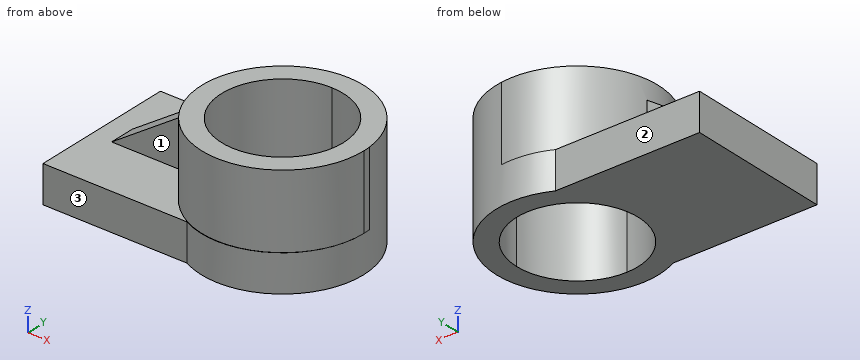
from build123d import *

# Parameters (mm, degrees)
F1_DEPTH = 25.4
F2_DEPTH = 76.2
F4_DEPTH = 50.8
F6_DEPTH = 38.1
F9_DEPTH = 50.8


with BuildPart() as f1:
    # F0 (on Top) → F1 (new body)
    with BuildSketch(Plane.XY):
        with BuildLine():
            ThreePointArc((36.7828311237, -49.6836304665), (6.3025091863, 0), (36.7828311237, 49.6836304665))
            Line((36.7828311237, 49.6836304665), (-62.0354041457, 49.6836304665))
            Line((-62.0354041457, 49.6836304665), (-62.0354041457, -49.6836304665))
            Line((-62.0354041457, -49.6836304665), (36.7828311237, -49.6836304665))
        make_face()
    extrude(amount=F1_DEPTH)

    # F0 (on Top) → F2 (join)
    with BuildSketch(Plane.XY):
        with BuildLine():
            Line((62.0354041457, 41.7620725768), (62.0354041457, 49.6836304665))
            Line((62.0354041457, 49.6836304665), (36.7828311237, 49.6836304665))
            ThreePointArc((36.7828311237, 49.6836304665), (6.3025091863, 0), (36.7828311237, -49.6836304665))
            Line((36.7828311237, -49.6836304665), (62.0354041457, -49.6836304665))
            Line((62.0354041457, -49.6836304665), (62.0354041457, -41.7620725768))
            ThreePointArc((62.0354041457, -41.7620725768), (20.2733315689, 0), (62.0354041457, 41.7620725768))
        make_face()
        with BuildLine():
            Line((36.7828311237, 49.6836304665), (62.0354041457, 49.6836304665))
            Line((62.0354041457, 49.6836304665), (62.0354041457, 41.7620725768))
            ThreePointArc((62.0354041457, 41.7620725768), (91.5656488612, 29.5302447155), (103.7974767226, 0))
            ThreePointArc((103.7974767226, 0), (91.5656488612, -29.5302447155), (62.0354041457, -41.7620725768))
            Line((62.0354041457, -41.7620725768), (62.0354041457, -49.6836304665))
            Line((62.0354041457, -49.6836304665), (36.7828311237, -49.6836304665))
            ThreePointArc((36.7828311237, -49.6836304665), (91.1794994385, -47.5055500981), (117.7682991051, 0))
            ThreePointArc((117.7682991051, 0), (91.1794994385, 47.5055500981), (36.7828311237, 49.6836304665))
        make_face()
        with BuildLine():
            ThreePointArc((36.7828311237, -49.6836304665), (6.3025091863, 0), (36.7828311237, 49.6836304665))
            Line((36.7828311237, 49.6836304665), (-62.0354041457, 49.6836304665))
            Line((-62.0354041457, 49.6836304665), (-62.0354041457, -49.6836304665))
            Line((-62.0354041457, -49.6836304665), (36.7828311237, -49.6836304665))
        make_face()
    extrude(amount=F2_DEPTH)

    # F3 (on face) → F4 (cut)
    with BuildSketch(Plane.XY.offset(76.2)):
        with BuildLine():
            ThreePointArc((117.5399853374, 5.0395483226), (117.7039365392, 2.5789094219), (117.7586227951, 0.1134209896))
            ThreePointArc((117.7586227951, 0.1134209896), (20.3132089265, -36.5094395307), (69.5168613964, 55.2284652871))
            ThreePointArc((69.5168613964, 55.2284652871), (52.7273733531, 54.9501241429), (36.7828311237, 49.6836304665))
            Line((36.7828311237, 49.6836304665), (-62.0354041457, 49.6836304665))
            Line((-62.0354041457, 49.6836304665), (-62.0354041457, -49.6836304665))
            Line((-62.0354041457, -49.6836304665), (36.7828311237, -49.6836304665))
            ThreePointArc((36.7828311237, -49.6836304665), (93.2996420825, -46.1378695519), (117.5399853374, 5.0395483226))
        make_face()
    extrude(amount=-F4_DEPTH, mode=Mode.SUBTRACT)

    # F5 (on face) → F6 (join)
    with BuildSketch(Plane.XY.offset(25.4)):
        with BuildLine():
            ThreePointArc((7.2234576062, -8.5192370875), (6.5492578133, 0.1134209896), (7.2234576061, 8.7460790667))
            Line((7.2234576062, 8.7460790667), (-48.1677358464, 8.7460790667))
            Line((-48.1677358464, 8.7460790667), (-48.1677358464, -8.7460790667))
            Line((-48.1677358464, -8.7460790667), (7.2234576062, -8.7460790667))
            Line((7.2234576062, -8.7460790667), (7.2234576062, -8.5192370875))
        make_face()
    extrude(amount=F6_DEPTH)

    # F8 (on face) → F9 (cut)
    with BuildSketch(Plane.XZ.offset(8.7460790667)):
        Polygon((-48.1677358464, 63.5), (-48.1677358464, 25.4008052661), (7.095429115, 63.304014504), (7.2234576062, 63.4966630391), (7.2234576062, 63.5), align=None)
    extrude(amount=-F9_DEPTH, mode=Mode.SUBTRACT)


solid = f1.part
Here's how the part is built. I have some questions about the finished solid (model axes, mm). Face numbers are marked on the shaded views. A direction names the side the tool comes from. Round coordinates to 2 decimals unless told otherwise and drop trailing zeros. Order: outer loops, then holes, each group sorted by start corner. A loop starts at its lowest first (then second) coordinate and runs counter-clockwise, first axis right, second up. Notation, with made-up numbers: M 59.25,68.25 L 118.25,68.25 A27 ccw 118.25,98.25 Z; hole C 20.25,29 d5. An arc over 180 degrees is marked long. Return JSON: item names as keys, results as strings. Group by question number.
1. If we section it at D-D on x = -29: List the corners of the cut face in (y, z) for me.
2. Please list where these lines run through material, in increasing order: probe 1 along Y at (x, z) = (62.5, 41); probe 2 along Z at (x, y) = (-29, -46.5); probe 3 along Y at (x, z) = (-15, 47.5).
3. If we section it at A-A on x = 81: List the corners of the cut face in (y, z) for me.
4. If we section it at C-C on y = -30.5: List the corners of the cut face in (x, z) for me, then the cut area to 3 significant figures.
5. If we section it at B-B on z = 22: List the corners of the cut face in (x, y) for me.
6. I'm going to push flat-ended pins straight in: pin 1 Ø1.5 at (y, z) = (17.5, 17.5) entering from +X; pin 2 Ø20.5 at (x, z) = (-31, 15) entering from +Y; pin 3 Ø5 at (x, y) = (-39.5, 24) entering from +Z. Where does each tip first touch, or does it pass through?
7. On a 3-axis mill with a long thin cutter (end or side, diameter ignored), from which of +Z, -Z, +X, -X, +Y, -Y can I reach the whole of each face in a straight line? I mean the marked faces 1, 2 and 3. Say none if no direction works.
Reply:
{
 "1": {"outline": "M -49.68,0 L 49.68,0 L 49.68,25.4 L 8.75,25.4 L 8.75,38.55 L -8.75,38.55 L -8.75,25.4 L -49.68,25.4 Z"},
 "2": {"probe 1": "-55.49 to -41.76, 41.76 to 55.72", "probe 2": "0 to 25.4", "probe 3": "-8.75 to 8.75"},
 "3": {"outline": "M -52.41,0 L -37.21,0 L -37.21,76.2 L -52.2,76.2 L -52.2,25.4 L -52.41,25.4 Z; M 37.21,0 L 52.41,0 L 52.41,76.2 L 37.21,76.2 Z"},
 "4": {"outline": "M -62.04,0 L 33.51,0 L 33.51,76.2 L 15.74,76.2 L 15.74,25.4 L -62.04,25.4 Z; M 90.56,0 L 108.68,0 L 108.68,25.4 L 108.57,25.4 L 108.57,76.2 L 90.56,76.2 Z", "area": "4,700 mm^2"},
 "5": {"outline": "M -62.04,-49.68 L 36.78,-49.68 A55.73 ccw long 36.78,49.68 L -62.04,49.68 Z; hole C 62.04,0 d83.52"},
 "6": {"pin 1": "x = 115.19", "pin 2": "y = 49.68", "pin 3": "z = 25.4"},
 "7": {"face 1": "+Z, -X, -Y", "face 2": "+Z, -Z, -X, +Y", "face 3": "+Z, -Z, -X, -Y"}
}
